Could you check a few things on this model? Use its own coordinates, in mm. Face numbers are marked on the shaded views. A direction names the side the tool comes from. Give positions to 0.01 mm unless a question says otherwise; leave off trailing zeros. Loops run counter-clockwise (first coordinate to the right, second up) from the corner with the lowest first, then second, coordinate; pieces in that order, holes last. Notation, with made-up numbers: M 4.25,68 L 28.25,68 A31 ccw 28.25,105 Z; hole C -25,-39.5 d7. An arc over 180 degrees is marked long. Answer in a Markdown table with one row per item. Add a question column.
1. If we section it at D-D on z = 10: Count the separate pieces of the cut face and the enclosed holes in it, then the cut area to 3 significant figures.
2. If we section it at C-C on y = -12.25: List the corners of the cut face in (x, z) for me.
3. Which directions (+Z, -Z, +X, -X, +Y, -Y) give clear straight access to the entire face, cutting with the end or side of a thin tool? Please do the marked faces 1, 2, 3, 4 and 5.
4. If we section it at B-B on x = 0: List the corners of the cut face in (y, z) for me.
5. I'm going to push flat-ended pins straight in: pin 1 Ø2 at (x, z) = (16.5, 2) entering from +Y; pin 2 Ø8 at (x, z) = (-41.5, 3) entering from -Y; pin 3 Ø6 at (x, y) = (37.5, -9) entering from +Z; pin 4 Ø5 at (x, z) = (-22.5, -2) entering from +Y. Where does each tip first touch, or does it pass through?
6. I need wall thicknesses on line 1 along Y through (x, z) = (57.95, 10); line 2 along X through (y, z) = (-5.2, 0); line 3 along Y through (x, z) = (-36.5, -2). Which ranges of each line are inside material? Lowest first, please. Write a range as from..to.
7. If we section it at A-A on z = 0: List the corners of the cut face in (x, y) for me, then the cut area to 3 significant figures.
8. Thinking about a two-plate mould opening in X: for the marked faces 6, 7 and 8, which applies, released by +X, released by -X, zero draft, split by the parting line, or undercut?
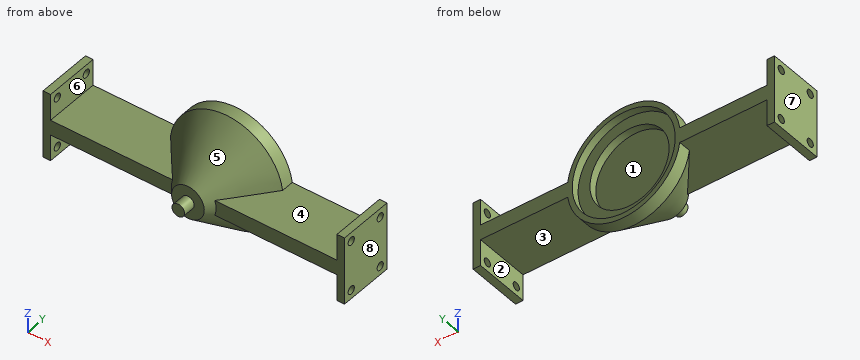
```python
from build123d import *

# Parameters (mm, degrees)
SKETCH1_R    = 22.5
BASE_DEPTH   = 50
SKETCH3_R    = 20.5
INSET_DEPTH  = 3
SKETCH11_R   = 15.75
INSET2_DEPTH = 3
PAD_START    = 60
SKETCH4_W    = 27
SKETCH4_H    = 22
SKETCH4_R    = 1.6
PAD_DEPTH    = 3
RIB_REACH    = 89.901
SKETCH5_W    = 6
SKETCH5_H    = 22
PAD2_START   = -60
SKETCH4_2_W  = 27
SKETCH4_2_H  = 22
SKETCH4_2_R  = 1.6
PAD2_DEPTH   = 3
RIB2_REACH   = 124.863
SKETCH8_W    = 6
SKETCH8_H    = 22


with BuildPart() as part:
    # Sketch1 → Base (new body)
    with BuildSketch(Plane(origin=(0, 0, 0), x_dir=(1, 0, 0), z_dir=(0, 1, 0))):
        with Locations(Location((0, 0, 0), (0, 0, 270))):
            Circle(SKETCH1_R)
    extrude(amount=-BASE_DEPTH)

    # Sketch2 → Cone (revolve, cut)
    with BuildSketch(Plane(origin=(0, 0, 0), x_dir=(0, 0, -1), z_dir=(1, 0, 0)), mode=Mode.PRIVATE) as cone_sk:
        Polygon((33.595146004, -5), (33.595146004, -56.971439611), (0, -56.971439611), (0, -30), (2.5, -30), (2.5, -25), (6.5, -25), (22.5, -5), align=None)
    revolve(cone_sk.sketch.rotate(Axis((0, 0, 0), (0, -1, 0)), 180), axis=Axis((0, 0, 0), (0, -1, 0)), mode=Mode.SUBTRACT)

    # Sketch3 → Inset (cut)
    with BuildSketch(Plane(origin=(0, 0, 0), x_dir=(1, 0, 0), z_dir=(0, 1, 0))):
        with Locations(Location((0, 0, 0), (0, 0, 270))):
            Circle(SKETCH3_R)
    extrude(amount=-INSET_DEPTH, mode=Mode.SUBTRACT)

    # Sketch11 → Inset2 (cut)
    with BuildSketch(Plane(origin=(0, -3, 0), x_dir=(1, 0, 0), z_dir=(0, 1, 0))):
        with Locations(Location((0, 0, 0), (0, 0, 270))):
            Circle(SKETCH11_R)
    extrude(amount=-INSET2_DEPTH, mode=Mode.SUBTRACT)

    # Sketch5 → Rib (add, up to next)
    with BuildSketch(Plane.ZY.offset(-57), mode=Mode.PRIVATE) as rib_sk1:
        with Locations((0, -11)):
            Rectangle(SKETCH5_W, SKETCH5_H)
    rib_tool1 = extrude(rib_sk1.sketch, amount=RIB_REACH, mode=Mode.PRIVATE) - part.part


with BuildPart() as body_2:
    # Sketch4 → Pad (new body)
    with BuildSketch(Plane(origin=(0, 0, 0), x_dir=(0, 0, -1), z_dir=(1, 0, 0)).offset(PAD_START)):
        with Locations((0, -11)):
            Rectangle(SKETCH4_W, SKETCH4_H)
        with Locations((-10, -3.5)):
            Circle(SKETCH4_R, mode=Mode.SUBTRACT)
        with Locations(Location((-10, -18.5, 0), (0, 0, 180))):
            Circle(SKETCH4_R, mode=Mode.SUBTRACT)
        with Locations((10, -18.5)):
            Circle(SKETCH4_R, mode=Mode.SUBTRACT)
        with Locations(Location((10, -3.5, 0), (0, 0, 180))):
            Circle(SKETCH4_R, mode=Mode.SUBTRACT)
    extrude(amount=-PAD_DEPTH)


with BuildPart() as part_1:
    add(part.part)

    add(body_2.part)  # Rib merges body 2
    add(rib_tool1.solids().sort_by_distance((57, -11, 0))[0])

    # Sketch8 → Rib2 (add, up to next)
    with BuildSketch(Plane(origin=(-57, 0, 0), x_dir=(0, 0, -1), z_dir=(1, 0, 0)), mode=Mode.PRIVATE) as rib2_sk1:
        with Locations((0, -11)):
            Rectangle(SKETCH8_W, SKETCH8_H)
    rib2_tool1 = extrude(rib2_sk1.sketch, amount=RIB2_REACH, mode=Mode.PRIVATE) - part_1.part


with BuildPart() as body_2_2:
    # Sketch4_2 → Pad2 (new body)
    with BuildSketch(Plane(origin=(0, 0, 0), x_dir=(0, 0, -1), z_dir=(1, 0, 0)).offset(PAD2_START)):
        with Locations((0, -11)):
            Rectangle(SKETCH4_2_W, SKETCH4_2_H)
        with Locations((-10, -3.5)):
            Circle(SKETCH4_2_R, mode=Mode.SUBTRACT)
        with Locations(Location((-10, -18.5, 0), (0, 0, 180))):
            Circle(SKETCH4_2_R, mode=Mode.SUBTRACT)
        with Locations((10, -18.5)):
            Circle(SKETCH4_2_R, mode=Mode.SUBTRACT)
        with Locations(Location((10, -3.5, 0), (0, 0, 180))):
            Circle(SKETCH4_2_R, mode=Mode.SUBTRACT)
    extrude(amount=PAD2_DEPTH)


with BuildPart() as part_2:
    add(part_1.part)

    add(body_2_2.part)  # Rib2 merges body 2 2
    add(rib2_tool1.solids().sort_by_distance((-57, -11, 0))[0])


solid = part_2.part
```
Results:
| question | item | result |
|---|---|---|
| 1 | separate pieces | 7 |
| 1 | enclosed holes | 0 |
| 1 | area | 500 mm2 |
| 2 | outline | M -60,-13.5 L -57,-13.5 L -57,-3 L -16.43,-3 A16.7 ccw 16.43,-3 L 57,-3 L 57,-13.5 L 60,-13.5 L 60,13.5 L 57,13.5 L 57,3 L 16.43,3 A16.7 ccw -16.43,3 L -57,3 L -57,13.5 L -60,13.5 Z |
| 3 | face 1 | +Y |
| 3 | face 2 | -Z, +Y, -Y |
| 3 | face 3 | -Z, -Y |
| 3 | face 4 | +Z, -Y |
| 3 | face 5 | -Y |
| 4 | outline | M -30,-2.5 L -25,-2.5 L -25,-6.5 L -5,-22.5 L 0,-22.5 L 0,-20.5 L -3,-20.5 L -3,-15.75 L -6,-15.75 L -6,15.75 L -3,15.75 L -3,20.5 L 0,20.5 L 0,22.5 L -5,22.5 L -25,6.5 L -25,2.5 L -30,2.5 Z |
| 5 | pin 1 | y = -3 |
| 5 | pin 2 | y = -22 |
| 5 | pin 3 | z = 3 |
| 5 | pin 4 | y = 0 |
| 6 | line 1 | -22..-20.1, -16.9..-5.1, -1.9..0 |
| 6 | line 2 | -60..-15.75, 15.75..60 |
| 6 | line 3 | -22..0 |
| 7 | outline | M -60,-22 L -8.9,-22 L -6.5,-25 L -2.5,-25 L -2.5,-30 L 2.5,-30 L 2.5,-25 L 6.5,-25 L 8.9,-22 L 60,-22 L 60,0 L 20.5,0 L 20.5,-3 L 15.75,-3 L 15.75,-6 L -15.75,-6 L -15.75,-3 L -20.5,-3 L -20.5,0 L -60,0 Z |
| 7 | area | 2,490 mm2 |
| 8 | face 6 | undercut |
| 8 | face 7 | released by -X |
| 8 | face 8 | released by +X |
